Verification items for the finished model (mm, model axes). Give positions to 0.01 mm unless a question says otherwise; leave off trailing zeros. Loops run counter-clockwise (first coordinate to the right, second up) from the corner with the lowest first, then second, coordinate; pieces in that order, holes last. Notation, with made-up numbers: (43, 47.5) - (79, 47.5) arc R12 ccw to (79, 59.5) - close; hole circle Ø10 at (36.5, 70.5). An arc over 180 degrees is marked (long way). Use one line per item in the form item = value.
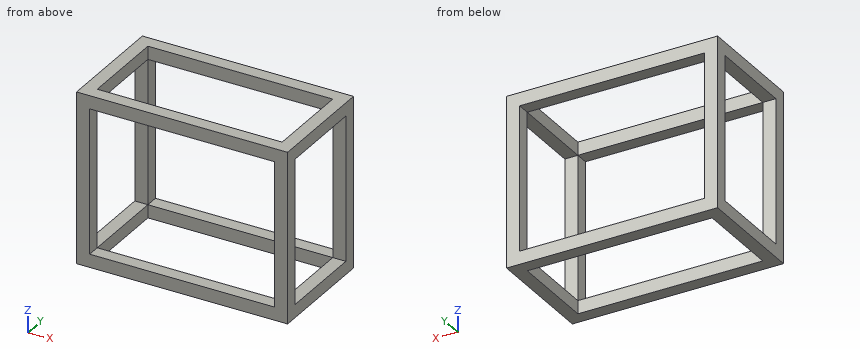
Autodesk Inventor part; units mm, degrees
ref_plane "YZ Plane" through (0, 0, 0) normal (1, 0, 0) x (0, 1, 0)
ref_plane "XZ Plane" through (0, 0, 0) normal (0, 1, 0) x (-1, 0, 0)
ref_plane "XY Plane" through (0, 0, 0) normal (0, 0, 1) x (1, 0, 0)
sketch "Sketch1" plane through (0, 0, 0) normal (0, 0, 1) x (1, 0, 0)
  line L0 (0, 0) -> (322.448, 0)
  line L1 (322.448, 0) -> (322.448, 173.35)
  line L2 (322.448, 173.35) -> (0, 173.35)
  line L3 (0, 173.35) -> (0, 0)
  dimension "d0" = 322.448
  dimension "d1" = 173.35
extrude "Extrusion1" add sketch "Sketch1" along normal blind 260.725
sketch "Sketch2" plane through (0, 0, 260.725) normal (0, 0, 1) x (1, 0, 0)
  line L0 (20, 153.35) -> (302.448, 153.35)
  line L1 (302.448, 153.35) -> (302.448, 20)
  line L2 (302.448, 20) -> (20, 20)
  line L3 (20, 20) -> (20, 153.35)
  line L4 (322.448, 173.35) -> (0, 173.35)
  line L5 (0, 173.35) -> (0, 0)
  line L6 (0, 0) -> (322.448, 0)
  line L7 (322.448, 0) -> (322.448, 173.35)
  dimension "d4" = 20
  dimension "d5" = 20
  dimension "d6" = 20
  dimension "d7" = 20
extrude "Extrusion2" cut sketch "Sketch2" against normal blind 900 contours L0 L1 L2 L3
sketch "Sketch3" plane through (322.448, 0, 0) normal (1, 0, 0) x (0, 0, -1)
  line L0 (-240.725, 153.35) -> (-20, 153.35)
  line L1 (-20, 153.35) -> (-20, 20)
  line L2 (-20, 20) -> (-240.725, 20)
  line L3 (-240.725, 20) -> (-240.725, 153.35)
  line L4 (0, 173.35) -> (-260.725, 173.35)
  line L5 (-260.725, 0) -> (-260.725, 173.35)
  line L6 (0, 0) -> (-260.725, 0)
  line L7 (0, 0) -> (0, 173.35)
  dimension "d10" = 20
  dimension "d11" = 20
  dimension "d12" = 20
  dimension "d13" = 20
extrude "Extrusion3" cut sketch "Sketch3" against normal blind 900 contours L0 L1 L2 L3
sketch "Sketch4" plane through (0, 173.35, 0) normal (0, 1, 0) x (1, 0, 0)
  line L0 (20, -20) -> (302.448, -20)
  line L1 (302.448, -20) -> (302.448, -240.725)
  line L2 (302.448, -240.725) -> (20, -240.725)
  line L3 (20, -240.725) -> (20, -20)
  line L4 (322.448, 0) -> (0, 0)
  line L5 (0, 0) -> (0, -260.725)
  line L6 (322.448, 0) -> (322.448, -260.725)
  line L7 (322.448, -260.725) -> (0, -260.725)
  dimension "d16" = 20
  dimension "d17" = 20
  dimension "d18" = 20
  dimension "d19" = 20
extrude "Extrusion4" cut sketch "Sketch4" against normal blind 900 contours L0 L1 L2 L3
properties part number "Turning motor housing"
1. Scan lines: probe 1 along X at (y, z) = (35.5, 247); probe 2 along Y at (x, z) = (125.5, 13); probe 3 along Z at (x, y) = (203.5, 14) (3 decimals). Record each from-to range of solid material in increasing order.
Result set:
probe_1 = 0 to 20, 302.45 to 322.45
probe_2 = 0 to 20, 153.35 to 173.35
probe_3 = 0 to 20, 240.725 to 260.725
2. Section check A-A, the plane z = 202. Record the cut outline in (x, y).
Result set:
outline = (0, 0) - (20, 0) - (20, 20) - (0, 20) - close; (0, 153.35) - (20, 153.35) - (20, 173.35) - (0, 173.35) - close; (302.45, 0) - (322.45, 0) - (322.45, 20) - (302.45, 20) - close; (302.45, 153.35) - (322.45, 153.35) - (322.45, 173.35) - (302.45, 173.35) - close
3. Section check B-B, the plane y = 117. Record the cut outline in (x, z) (3 decimals), then the cut area to 3 significant figures.
Result set:
outline = (0, 0) - (20, 0) - (20, 20) - (0, 20) - close; (0, 240.725) - (20, 240.725) - (20, 260.725) - (0, 260.725) - close; (302.448, 0) - (322.448, 0) - (322.448, 20) - (302.448, 20) - close; (302.448, 240.725) - (322.448, 240.725) - (322.448, 260.725) - (302.448, 260.725) - close
area = 1,600 mm²
